Build history of the part. All positions in model axes, mm. Give positions to 0.01 mm unless a question says otherwise; leave off trailing zeros. Write each loop counter-clockwise with the first axis right and the second up, starting at its lowest first coordinate (ties: lowest second). Pieces come first, ordered by that corner, then holes. Notation, with made-up numbers: (31, 61.25) -> (82, 61.25) arc R11 cw to (82, 80.25) -> close; hole circle Ø3 at (-40, -19). An arc over 180 degrees is marked (long way). One line per question, with ' | ' between items. Start each with the question number.
(1) Band-saw the part on D-D, the plane x = 105. Give the cut face in (y, z).
(2) Pull direction Y, two halves, no side cores. Call faces 1 (the cylindrical face through (35.607, 61.227, 1.479)), 2 (the cylindrical face through (-64.297, 93.986, 1.479)), 3 (the flat face through (90, 26, 0)): released by +Y, released by -Y, zero draft, split by the parting line, or undercut.
(3) Band-saw the part on B-B, the plane y = 50. Give the cut face in (x, z), and give its area (3 significant figures).
(4) Band-saw the part on C-C, the plane z = 2.45. Count the separate pieces of the cut face and the enclosed holes in it, and give its area (3 significant figures).
(5) Pin check, flat tips, straight feed: P1, Ø1, axis at x = 192.5, z = 0.5, coming from the -Y side; P2, Ø1.5, axis at x = 188.5, z = 1, coming from the +Y side. Stop position of each tip, or through.
(6) Drill centre lines: probe 1 along Y at (x, z) = (320, 1.2); probe 2 along X at (y, z) = (9, 1.1); probe 3 along X at (y, z) = (44.5, 1). Where is each one in solid material? Low to high. Write a range as from..to.
(7) Band-saw the part on A-A, the plane x = 222. Give the cut face in (y, z).
Autodesk Inventor part; units mm, degrees
ref_plane "YZ Plane" through (0, 0, 0) normal (1, 0, 0) x (0, 1, 0)
ref_plane "XZ Plane" through (0, 0, 0) normal (0, 1, 0) x (-1, 0, 0)
ref_plane "XY Plane" through (0, 0, 0) normal (0, 0, 1) x (1, 0, 0)
sketch "Sketch1" plane through (0, 0, 0) normal (0, 0, 1) x (1, 0, 0)
  line L0 (0, 0) -> (350, 0)
  line L1 (350, 0) -> (350, 70)
  line L2 (350, 70) -> (0, 70)
  line L3 (0, 70) -> (0, 0)
  circle A0 centre (22.6, 65.5) radius 1.55
  circle A1 centre (22.6, 34.5) radius 1.55
  circle A2 centre (53.6, 65.5) radius 1.55
  circle A3 centre (53.6, 34.5) radius 1.55
  circle A4 centre (38.1, 50) radius 11.5
  line L4 (170, 18.1) -> (290, 18.1)
  line L5 (290, 18.1) -> (290, 15)
  line L6 (290, 15) -> (170, 15)
  line L7 (170, 15) -> (170, 18.1)
  line L8 (0, 70) -> (89.6145, 70)
  line L9 (250, 70) -> (287.051, 70)
  line L10 (250, 70) -> (270, 70)
  line L11 (270, 70) -> (270, 73)
  line L12 (270, 73) -> (250, 73)
  line L13 (250, 73) -> (250, 70)
  line L14 (310, 70) -> (310, 73)
  line L15 (310, 73) -> (290, 73)
  line L16 (290, 73) -> (290, 70)
  line L17 (290, 70) -> (327.051, 70)
  line L18 (290, 70) -> (310, 70)
  line L19 (350, 70) -> (350, 73)
  line L20 (350, 73) -> (330, 73)
  line L21 (330, 73) -> (330, 70)
  line L22 (330, 70) -> (367.051, 70)
  line L23 (330, 70) -> (350, 70)
  line L24 (8.1, 35) -> (5, 35)
  line L25 (5, 35) -> (5, 65)
  line L26 (5, 65) -> (8.1, 65)
  line L27 (8.1, 65) -> (8.1, 35)
  line L28 (8.1, 35) -> (5, 65) construction
  line L29 (5, 35) -> (8.1, 65) construction
  circle A5 centre (335, 10) radius 2.05
  circle A6 centre (320, 10) radius 2.05
  circle A7 centre (335, 60) radius 2.05
  circle A8 centre (320, 60) radius 2.05
  circle A9 centre (305, 60) radius 2.05
  circle A10 centre (305, 10) radius 2.05
  circle A11 centre (160, 10) radius 2.05
  circle A12 centre (145, 10) radius 2.05
  circle A13 centre (160, 60) radius 2.05
  circle A14 centre (145, 60) radius 2.05
  line L30 (325, 18.1) -> (345, 18.1)
  line L31 (345, 18.1) -> (345, 15)
  line L32 (345, 15) -> (325, 15)
  line L33 (325, 15) -> (325, 18.1)
  line L34 (0, 70) -> (100, 70)
  line L35 (100, 70) -> (100, 100)
  line L36 (100, 100) -> (0, 100)
  line L37 (0, 100) -> (0, 70)
  point P0 (6.55, 50)
  point P1 (5, 50)
  point P2 (8.1, 50)
  point P3 (170, 16.55)
  point P4 (290, 70)
  point P5 (100, 70)
  dimension "d1" = 3.1
  dimension "d2" = 3.1
  dimension "d3" = 3.1
  dimension "d4" = 3.1
  dimension "d5" = 31
  dimension "d7" = 23
  dimension "d8" = 15.5
  dimension "d9" = 15.5
  dimension "d10" = 70
  dimension "d11" = 31
  dimension "d12" = 3.1
  dimension "d13" = 50
  dimension "d46" = 20
  dimension "d47" = 3
  dimension "d48" = 20
  dimension "d49" = 3
  dimension "d50" = 20
  dimension "d51" = 3
  dimension "d52" = 20
  dimension "d53" = 20
  dimension "d54" = 350
  dimension "d55" = 3.1
  dimension "d56" = 5
  dimension "d57" = 15
  dimension "d58" = 30
  dimension "d59" = 120
  dimension "d63" = 4.1
  dimension "d64" = 4.1
  dimension "d65" = 4.1
  dimension "d66" = 4.1
  dimension "d67" = 4.1
  dimension "d68" = 4.1
  dimension "d69" = 15
  dimension "d70" = 15
  dimension "d71" = 10
  dimension "d72" = 10
  dimension "d73" = 15
  dimension "d79" = 4.1
  dimension "d80" = 4.1
  dimension "d81" = 4.1
  dimension "d82" = 4.1
  dimension "d85" = 15
  dimension "d87" = 10
  dimension "d88" = 10
  dimension "d89" = 10
  dimension "d90" = 60
  dimension "d91" = 5
  dimension "d92" = 20
  dimension "d93" = 15
  dimension "d94" = 100
  dimension "d95" = 30
extrude "Extrusion1" add sketch "Sketch1" along normal blind 3 contours L3 L2 L1 L0 | L37 L36 L35 L2 | L2 L21 L20 L19
sketch "Sketch3" plane through (0, 0, 3) normal (0, 0, 1) x (1, 0, 0)
  line L0 (0, 100) -> (0, 0)
  line L1 (0, 100) -> (-70, 100)
  line L2 (-70, 100) -> (-70, -50)
  line L3 (-70, -50) -> (100, -50)
  line L4 (100, -50) -> (100, 0)
  line L5 (0, 0) -> (350, 0)
  dimension "d99" = 70
  dimension "d100" = 150
  dimension "d101" = 170
extrude "Extrusion3" add sketch "Sketch3" against normal blind 3
fillet "Fillet1" radius 20 1 edges at (-70, 100, 1.5)
properties part number "Sideboard"
Results:
1) outline: (0, 0) -> (70, 0) -> (70, 3) -> (0, 3) -> close
2) face 1: undercut | face 2: released by +Y | face 3: zero draft
3) outline: (-70, 0) -> (5, 0) -> (5, 3) -> (-70, 3) -> close; (8.1, 0) -> (26.6, 0) -> (26.6, 3) -> (8.1, 3) -> close; (49.6, 0) -> (350, 0) -> (350, 3) -> (49.6, 3) -> close | area: 1,180 mm²
4) separate pieces: 1 | enclosed holes: 18 | area: 41,900 mm²
5) P1: stops at y = 0 | P2: stops at y = 70
6) probe 1: y = 0..7.95, 12.05..57.95, 62.05..70 | probe 2: x = -70..143.21, 146.79..158.21, 161.79..303.21, 306.79..318.21, 321.79..333.21, 336.79..350 | probe 3: x = -70..5, 8.1..28, 48.2..350
7) outline: (0, 0) -> (15, 0) -> (15, 3) -> (0, 3) -> close; (18.1, 0) -> (70, 0) -> (70, 3) -> (18.1, 3) -> close
